from build123d import *

# Parameters (mm, degrees)
BOSS_EXTRUDE1_DEPTH            = 30
CUT_EXTRUDE1_DEPTH             = 282.336097933
CHAMFER1_SIZE                  = 5
CBORE_FOR_M4_SHCS2_D           = 4.5
CBORE_FOR_M4_SHCS2_CBORE_D     = 8
CBORE_FOR_M4_SHCS2_CBORE_DEPTH = 4
CBORE_FOR_M4_SHCS1_D           = 4.5
CBORE_FOR_M4_SHCS1_CBORE_D     = 8
CBORE_FOR_M4_SHCS1_CBORE_DEPTH = 4
CUT_EXTRUDE2_DEPTH             = 25
SKETCH11_W                     = 27.5
SKETCH11_H                     = 47
CUT_EXTRUDE3_DEPTH             = 282.336097933
CBORE_FOR_M5_SHCS2_D           = 5.5
CBORE_FOR_M5_SHCS2_CBORE_D     = 10
CBORE_FOR_M5_SHCS2_CBORE_DEPTH = 5
M3X0_5_TAPPED_HOLE1_D          = 2.5
SKETCH21_W                     = 185
SKETCH21_H                     = 6.1
BOSS_EXTRUDE3_DEPTH            = 4
SKETCH22_W                     = 55
SKETCH22_H                     = 6.1
BOSS_EXTRUDE4_DEPTH            = 4
SKETCH23_W                     = 100
SKETCH23_H                     = 30
BOSS_EXTRUDE5_DEPTH            = 10
SKETCH24_W                     = 60
SKETCH24_H                     = 20
CUT_EXTRUDE4_DEPTH             = 10
CBORE_FOR_M5_SHCS3_D           = 5.5
CBORE_FOR_M5_SHCS3_CBORE_D     = 10
CBORE_FOR_M5_SHCS3_CBORE_DEPTH = 5
FILLET1_R                      = 5
CHAMFER2_SIZE                  = 0.5


with BuildPart() as part:
    # Sketch1 → Boss-Extrude1 (new body)
    with BuildSketch(Plane(origin=(0, 0, 0), x_dir=(1, 0, 0), z_dir=(0, 1, 0))):
        Polygon((245, 10), (50, 10), (50, 125), (100, 125), (100, 135), (0, 135), (0, 0), (245, 0), align=None)
    extrude(amount=BOSS_EXTRUDE1_DEPTH)

    # Sketch3 → Cut-Extrude1 (cut, through all)
    with BuildSketch(Plane.XZ):
        Polygon((50, 0), (0, -50), (0, 0), align=None)
    extrude(amount=-CUT_EXTRUDE1_DEPTH, mode=Mode.SUBTRACT)

    # Chamfer1
    chamfer1_edges = [part.edges().sort_by_distance(p)[0] for p in [
        (50, 15, -125),
        (50, 15, -10),
    ]]
    chamfer(chamfer1_edges, length=CHAMFER1_SIZE)

    # CBORE for M4 SHCS2 (through all)
    with Locations(Plane.XY):
        with Locations((240, 17.5), (90, 17.5)):
            CounterBoreHole(CBORE_FOR_M4_SHCS2_D / 2, CBORE_FOR_M4_SHCS2_CBORE_D / 2, CBORE_FOR_M4_SHCS2_CBORE_DEPTH)

    # CBORE for M4 SHCS1 (through all)
    with Locations(Plane(origin=(0, 0, -135), x_dir=(-1, 0, 0), z_dir=(0, 0, -1))):
        with Locations((-90, 17.5)):
            CounterBoreHole(CBORE_FOR_M4_SHCS1_D / 2, CBORE_FOR_M4_SHCS1_CBORE_D / 2, CBORE_FOR_M4_SHCS1_CBORE_DEPTH)

    # Sketch10 → Cut-Extrude2 (cut)
    with BuildSketch(Plane(origin=(0, 30, 0), x_dir=(1, 0, 0), z_dir=(0, 1, 0))):
        Polygon((55, 125), (10, 125), (10, 55), (50, 15), align=None)
    extrude(amount=-CUT_EXTRUDE2_DEPTH, mode=Mode.SUBTRACT)

    # Sketch11 → Cut-Extrude3 (cut, through all)
    with BuildSketch(Plane(origin=(0, 30, 0), x_dir=(1, 0, 0), z_dir=(0, 1, 0))):
        with Locations((23.75, 73.5)):
            Rectangle(SKETCH11_W, SKETCH11_H)
    extrude(amount=-CUT_EXTRUDE3_DEPTH, mode=Mode.SUBTRACT)

    # CBORE for M5 SHCS2 (through all)
    with Locations(Plane(origin=(10, 0, 0), x_dir=(0, 0, -1), z_dir=(1, 0, 0))):
        with Locations((115, 10)):
            CounterBoreHole(CBORE_FOR_M5_SHCS2_D / 2, CBORE_FOR_M5_SHCS2_CBORE_D / 2, CBORE_FOR_M5_SHCS2_CBORE_DEPTH)

    # M3x0.5 Tapped Hole1 (through all)
    with Locations(Plane(origin=(0, 0, 0), x_dir=(-1, 0, 0), z_dir=(0, -1, 0))):
        with Locations((-4, 73.5), (-43.5, 73.5)):
            Hole(M3X0_5_TAPPED_HOLE1_D / 2)

    # Sketch21 → Boss-Extrude3 (add)
    with BuildSketch(Plane.XY):
        with Locations((142.5, 10)):
            Rectangle(SKETCH21_W, SKETCH21_H)
    extrude(amount=BOSS_EXTRUDE3_DEPTH)

    # Sketch22 → Boss-Extrude4 (add)
    with BuildSketch(Plane.ZY):
        with Locations((-77.5, 10)):
            Rectangle(SKETCH22_W, SKETCH22_H)
    extrude(amount=BOSS_EXTRUDE4_DEPTH)

    # Sketch23 → Boss-Extrude5 (add)
    with BuildSketch(Plane(origin=(0, 30, 0), x_dir=(1, 0, 0), z_dir=(0, 1, 0))):
        with Locations((145, -5)):
            Rectangle(SKETCH23_W, SKETCH23_H)
    extrude(amount=-BOSS_EXTRUDE5_DEPTH)

    # Sketch24 → Cut-Extrude4 (cut)
    with BuildSketch(Plane.XZ.offset(-20)):
        with Locations((145, 10)):
            Rectangle(SKETCH24_W, SKETCH24_H)
    extrude(amount=-CUT_EXTRUDE4_DEPTH, mode=Mode.SUBTRACT)

    # CBORE for M5 SHCS3 (through all)
    with Locations(Plane(origin=(0, 30, 0), x_dir=(1, 0, 0), z_dir=(0, 1, 0))):
        with Locations((105, -10), (185, -10)):
            CounterBoreHole(CBORE_FOR_M5_SHCS3_D / 2, CBORE_FOR_M5_SHCS3_CBORE_D / 2, CBORE_FOR_M5_SHCS3_CBORE_DEPTH)

    # Fillet1
    # the kernel refuses this fillet: 5 mm, written as the material it adds along each edge
    with BuildSketch(Plane(origin=(195, 20, 0), x_dir=(1, 0, 0), z_dir=(0, 1, 0)), Plane(origin=(115, 20, 0), x_dir=(1, 0, 0), z_dir=(0, 1, 0))) as fillet1_piece_1:
        with BuildLine():
            CenterArc((FILLET1_R, -FILLET1_R), FILLET1_R, 90, 90)
            Line((0, -FILLET1_R), (0, 0))
            Line((0, 0), (FILLET1_R, 0))
        make_face()
    extrude(amount=10)
    with BuildSketch(Plane(origin=(175, 20, 0), x_dir=(-1, 0, 0), z_dir=(0, 1, 0))) as fillet1_piece_2:
        with BuildLine():
            CenterArc((FILLET1_R, FILLET1_R), FILLET1_R, 180, 90)
            Line((0, FILLET1_R), (0, 0))
            Line((0, 0), (FILLET1_R, 0))
        make_face()
    extrude(amount=10)
    with BuildSketch(Plane(origin=(95, 30, 0), x_dir=(-1, 0, 0), z_dir=(0, -1, 0))) as fillet1_piece_3_section:
        with BuildLine():
            CenterArc((FILLET1_R, -FILLET1_R), FILLET1_R, 90, 90)
            Line((0, -FILLET1_R), (0, 0))
            Line((0, 0), (FILLET1_R, 0))
        make_face()
    fillet1_piece_3 = extrude(amount=10, mode=Mode.PRIVATE)
    fillet1_piece_3 = fillet1_piece_3 - Plane(origin=(90, 17.5, 0), x_dir=(1, 0, 0), z_dir=(0, 0, 1)) * Cylinder(4, 40, mode=Mode.PRIVATE)
    add(fillet1_piece_3)
    # the kernel refuses this fillet: 5 mm, written as the material it takes off along each edge
    with BuildSketch(Plane(origin=(-4, -5.297448714, -105), x_dir=(0, 0, 1), z_dir=(0, 1, 0)), Plane(origin=(50, -5.297448714, 4), x_dir=(1, 0, 0), z_dir=(0, 1, 0))) as fillet1_2_piece_1:
        with BuildLine():
            CenterArc((4.898979486, 5), FILLET1_R, 191.536959033, 78.463040967)
            Line((0, 4), (0, 0))
            Line((0, 0), (4.898979486, 0))
        make_face()
    extrude(amount=30.594897428, mode=Mode.SUBTRACT)
    with BuildSketch(Plane(origin=(-4, 25.297448714, -50), x_dir=(1.0, 0, -1.5791812302263136e-12), z_dir=(0, -1, 0))) as fillet1_2_piece_2:
        with BuildLine():
            CenterArc((5, -4.898979486), FILLET1_R, 101.536959033, 78.463040967)
            Line((0, -4.898979486), (0, 0))
            Line((0, 0), (4, 0))
        make_face()
    extrude(amount=30.594897428, mode=Mode.SUBTRACT)
    with BuildSketch(Plane(origin=(195, 42.5, 20), x_dir=(0, 0, -1), z_dir=(0, -1, 0)), Plane(origin=(95, 42.5, 20), x_dir=(1, 0, 0), z_dir=(0, -1, 0))) as fillet1_2_piece_3:
        with BuildLine():
            CenterArc((FILLET1_R, -FILLET1_R), FILLET1_R, 90, 90)
            Line((0, -FILLET1_R), (0, 0))
            Line((0, 0), (FILLET1_R, 0))
        make_face()
    extrude(amount=35, mode=Mode.SUBTRACT)
    with BuildSketch(Plane(origin=(175, 7.5, 20), x_dir=(1, 0, 0), z_dir=(0, 1, 0)), Plane(origin=(115, 7.5, 20), x_dir=(0, 0, -1), z_dir=(0, 1, 0))) as fillet1_2_piece_4:
        with BuildLine():
            CenterArc((FILLET1_R, FILLET1_R), FILLET1_R, 180, 90)
            Line((0, FILLET1_R), (0, 0))
            Line((0, 0), (FILLET1_R, 0))
        make_face()
    extrude(amount=35, mode=Mode.SUBTRACT)
    with BuildSketch(Plane(origin=(100, -12.5, -135), x_dir=(0, 0, 1), z_dir=(0, 1, 0))) as fillet1_2_piece_5:
        with BuildLine():
            CenterArc((FILLET1_R, -FILLET1_R), FILLET1_R, 90, 90)
            Line((0, -FILLET1_R), (0, 0))
            Line((0, 0), (FILLET1_R, 0))
        make_face()
    extrude(amount=55, mode=Mode.SUBTRACT)

    # Chamfer2
    chamfer2_edges = [part.edges().sort_by_distance(p)[0] for p in [
        (150, 0, -10),
        (10, 0, -73.5),
        (37.5, 0, -73.5),
        (23.75, 0, -50),
        (23.75, 0, -97),
        (245, 0, -5),
        (0, 0, -92.5),
        (42.25, 0, -73.5),
        (2.75, 0, -73.5),
        (47.5, 0, -135),
        (98.535533906, 0, -133.535533906),
        (147.5, 0, 0),
        (25, 0, -25),
        (77.5, 0, -125),
        (50, 0, -67.5),
        (52.5, 0, -122.5),
        (52.5, 0, -12.5),
        (100, 0, -127.5),
    ]]
    chamfer(chamfer2_edges, length=CHAMFER2_SIZE)


solid = part.part
Source: CAD feature listing. Evaluate the final solid. Frame: model axes, mm. A direction names the side the tool comes from. Round coordinates to 2 decimals unless told otherwise and drop trailing zeros. Loops run counter-clockwise (first coordinate to the right, second up) from the corner with the lowest first, then second, coordinate; pieces in that order, holes last. Notation, with made-up numbers: M -32,-33 L -15,-33 A26 ccw -15,2 Z; hole C 87,68 d7. An arc over 180 degrees is marked long. Return JSON: item names as keys, results as strings. Group by question number.
1. Section query B-B on x = 185. Output: boundary loops of the cut face in (y, z), and give its area (3 significant figures).
2. Material intervals for line 1 along Z through (x, y) = (87, 28); line 2 along Y through (x, z) = (240, -8); line 3 along Z through (x, y) = (85, 11.5), sorted ascending. Write a range as from..to.
3. Section query A-A on y = 10. Output: boundary loops of the cut face in (x, z), and give its area (3 significant figures).
4. Section query C-C on z = -88.5. Output: boundary loops of the cut face in (x, y), and give its area (3 significant figures).
5. Pin query (flat end, axial travel): pin 1 (6.5 mm diameter, centred on y = 10, z = -115, fed in from +X); pin 2 (6 mm diameter, centred on y = 20.5, z = 1, fed in from -X); pin 3 (12 mm diameter, centred on x = 130.5, y = 19, fed in from -Z); pin 4 (15 mm diameter, centred on y = 14, z = -96.5, fed in from -X). Return the tip coordinate at first contact, or that it passes through.
6. Reachability of faces 1 (the face through (37.5, 3, -73)), 2 (the face through (106, 20, 5)), 3 (the face through (144, 10, 4)), 4 (the face through (176, 25, 18)), 5 (the face through (50, 3, -67)) from +Z, -Z, +X, -X, +Y, -Y: full face, straight path, thin tool, end or side. Return the list, or none.
7. Mould query, pull axis X, two halves, no side actions, for faces 6 (the face through (242.248, 17.599, -7.042)), 7 (the face through (-4, 10, -78)), 8 (the face through (188, 20, 10)), 9 (the face through (52.29, 0.25, -122.64)). Classes: released by +X, released by -X, zero draft, split by the parting line, or undercut.
8. Section query D-D on x = 125. Output: boundary loops of the cut face in (y, z), and give its area (3 significant figures).
Checks:
{
 "1": {"outline": "M 0,-9.5 L 0.5,-10 L 30,-10 L 30,5 L 25,5 L 25,7.25 L 20,7.25 L 20,0 L 13.05,0 L 13.05,4 L 6.95,4 L 6.95,0 L 0.5,0 L 0,-0.5 Z; M 20,12.75 L 25,12.75 L 25,15 L 30,15 L 30,20 L 20,20 Z", "area": "447 mm²"},
 "2": {"line 1": "z = -135..-125, -10..0", "line 2": "y = 0..15.25, 19.75..30", "line 3": "z = -135..-125, -10..4"},
 "3": {"outline": "M -4,-100.1 A5 ccw 0,-105 L 0,-112.25 L 5,-112.25 L 5,-110 L 10,-110 L 10,-50 L 15,-50 L 55,-10 L 245,-10 L 245,0 L 235,0 L 235,4 L 54.9,4 A5 ccw 50,0 L 0,-50 A5 ccw -4,-54.9 Z; M 0,-135 L 95,-135 A5 ccw 100,-130 L 100,-125 L 10,-125 L 10,-120 L 5,-120 L 5,-117.75 L 0,-117.75 Z; hole C 4,-73.5 d2.5", "area": "5,210 mm²"},
 "4": {"outline": "M -4,6.95 L 0,6.95 L 0,0.5 L 0.5,0 L 9.5,0 L 10,0.5 L 10,30 L 0,30 L 0,13.05 L -4,13.05 Z; M 37.5,0.5 L 38,0 L 49.5,0 L 50,0.5 L 50,5 L 37.5,5 Z", "area": "386 mm²"},
 "5": {"pin 1": "stops at x = 5", "pin 2": "stops at x = 48", "pin 3": "stops at z = -10", "pin 4": "stops at x = -4"},
 "6": {"face 1": "+Y, -Y", "face 2": "+Z, +X, -X", "face 3": "+Z, +X, -X, -Y", "face 4": "+Z, +Y, -Y", "face 5": "+X, +Y, -Y"},
 "7": {"face 6": "undercut", "face 7": "released by -X", "face 8": "zero draft", "face 9": "released by +X"},
 "8": {"outline": "M 0,-9.5 L 0.5,-10 L 30,-10 L 30,0 L 13.05,0 L 13.05,4 L 6.95,4 L 6.95,0 L 0.5,0 L 0,-0.5 Z", "area": "324 mm²"}
}
